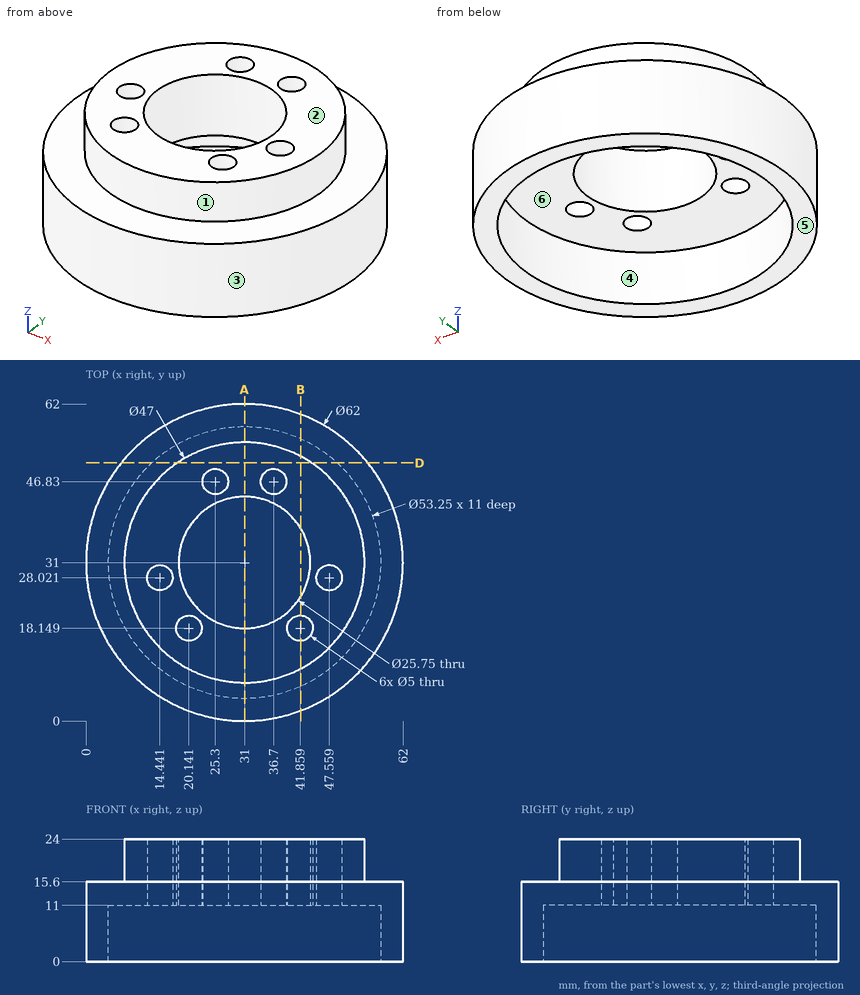
Study the drawing (mm; zero at the part's minimum x, y, z) and answer. A direction names the side the tool comes from. Round coordinates to 2 decimals unless told otherwise and drop trailing zeros. Loops run counter-clockwise (first coordinate to the right, second up) from the corner with the lowest first, then second, coordinate; pieces in that order, holes last. Notation, with made-up numbers: M 15.25,77 L 68.25,77 A23 ccw 68.25,111 Z; hole C 62,55.25 d2. An arc over 180 degrees is marked long. One line per question, with ' | ' between items.
Q1. Find section A-A, the plane x = 31. Give the vertices of the cut face in (y, z) (1 decimal).
Conclusion:
outline: M 0,0 L 4.4,0 L 4.4,11 L 18.1,11 L 18.1,24 L 7.5,24 L 7.5,15.6 L 0,15.6 Z; M 43.9,11 L 57.6,11 L 57.6,0 L 62,0 L 62,15.6 L 54.5,15.6 L 54.5,24 L 43.9,24 Z
Q2. Find section B-B, the plane x = 42. Give the vertices of the cut face in (y, z) (1 decimal).
Conclusion:
outline: M 2,0 L 6.8,0 L 6.8,11 L 15.7,11 L 15.7,24 L 10.2,24 L 10.2,15.6 L 2,15.6 Z; M 20.6,11 L 24.3,11 L 24.3,24 L 20.6,24 Z; M 37.7,11 L 55.2,11 L 55.2,0 L 60,0 L 60,15.6 L 51.8,15.6 L 51.8,24 L 37.7,24 Z
Q3. A tool of negligible diameter and unlimited length cuts with its end or side. For the marked faces 1 and 2, from which of +Z, -Z, +X, -X, +Y, -Y can it reach the whole face along a straight path? Write none if from no direction.
Conclusion:
face 1: +Z | face 2: +Z, +X, -X, +Y, -Y
Q4. Each of these flat-tipped pins is pushed along its axis until it touches: pin 1 Ø1.5 at (y, z) = (41.5, 21.5) entering from +X; pin 2 Ø4 at (x, y) = (14.44, 28.02) entering from -Z; pin 3 Ø8 at (y, z) = (49, 13) entering from +X; pin 4 Ø2 at (x, z) = (26, 20) entering from +Y. Where does it stop, or does it pass through?
Conclusion:
pin 1: stops at x = 52.38 | pin 2: passes through | pin 3: stops at x = 58.66 | pin 4: stops at y = 54.16
Q5. The mould has two halves that part along X. Classify the marked faces 3, 4, 5 and 6: +X half, -X half, draft (parallel to the pull), parting line (faces both ways), or undercut.
Conclusion:
face 3: parting line | face 4: undercut | face 5: draft | face 6: undercut
Q6. Find section D-D, the plane y = 50.5. Give the vertices of the cut face in (x, z) (1 decimal).
Conclusion:
outline: M 6.9,0 L 12.9,0 L 12.9,11 L 49.1,11 L 49.1,0 L 55.1,0 L 55.1,15.6 L 44.1,15.6 L 44.1,24 L 17.9,24 L 17.9,15.6 L 6.9,15.6 Z
Q7. Consider line 1 along X through (y, z) = (26, 17.25) (1 decimal); line 2 along Y through (x, z) = (31, 21.5) (1 decimal); line 3 along Z through (x, y) = (31, 55). Determine where each line is inside the solid, lowest interval first. Write a range as from..to.
Conclusion:
line 1: x = 8..13, 15.9..19.1, 42.9..46.1, 49..54 | line 2: y = 7.5..18.1, 43.9..54.5 | line 3: z = 11..15.6
